Verification items for the finished model (mm, model axes). Face numbers are marked on the shaded views. A direction names the side the tool comes from. Coordinates: 2 decimals unless noted, no trailing zeros. Write each loop counter-clockwise with the first axis right and the second up, starting at its lowest first coordinate (ties: lowest second). Pieces come first, ordered by that corner, then holes. Notation, with made-up numbers: (38, -4) -> (50, -4) arc R25 ccw to (50, 8) -> close; hole circle Ø4 at (48.25, 9). An arc over 180 degrees is marked (long way). Write each question's results on one line, items separated by ' | '. Start each with the question number.
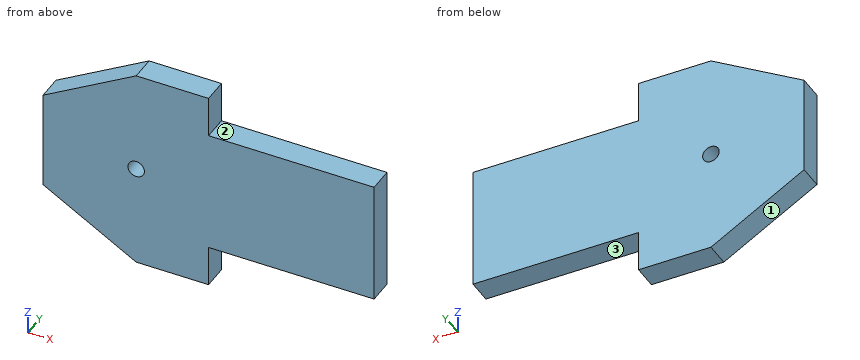
from build123d import *

# Parameters (mm, degrees)
BOSS_EXTRUDE1_DEPTH = 3
SKETCH2_R           = 1
CUT_EXTRUDE1_DEPTH  = 33


with BuildPart() as part:
    # Sketch1 → Boss-Extrude1 (new body)
    with BuildSketch(Plane(origin=(0, 0, 0), x_dir=(1, 0, 0), z_dir=(0, 1, 0))):
        Polygon((-10, 7.5), (-10, 12.5), (-18.741669751, 12.5), (-30, 6), (-30, -6), (-18.741669751, -12.5), (-10, -12.5), (-10, -7.5), (10, -7.5), (10, 7.5), align=None)
    extrude(amount=BOSS_EXTRUDE1_DEPTH)

    # Sketch2 → Cut-Extrude1 (cut)
    with BuildSketch(Plane(origin=(0, 3, 0), x_dir=(1, 0, 0), z_dir=(0, 1, 0))):
        with Locations(Location((-18.741669751, 0, 0), (0, 0, 270))):
            Circle(SKETCH2_R)
    extrude(amount=-CUT_EXTRUDE1_DEPTH, mode=Mode.SUBTRACT)


solid = part.part
1. Depth check by flat-ended pin: pin 1 Ø1.5 at (x, z) = (-5.5, -8.5) entering from +Y; pin 2 Ø1.5 at (y, z) = (1, -9.5) entering from +X; pin 3 Ø0.9 at (x, y) = (1.5, 2) entering from -Z. Enter the tip coordinate at first touch or a pass-through.
2. Material ranges on probe 1 along X at (y, z) = (1.3, 0); probe 2 along Z at (x, y) = (6.5, 1.2); probe 3 along X at (y, z) = (2.4, 8.75), recorded low to high. Write a range as from..to.
3. Sectioned sample at C-C on x = 4.5. Record the cut outline in (y, z), plus the area to 3 significant figures.
4. Sectioned sample at A-A on y = 1.7. Record the cut outline in (x, z), plus the area to 3 significant figures.
5. Tool access check on the marked faces 1, 2 and 3. Record the directions out of +Z, -Z, +X, -X, +Y, -Y that give a thin tool (end or side, any length) a straight path to the whole face; none if there is none.
6. Sectioned sample at D-D on x = -21. Record the cut outline in (y, z).
7. Sectioned sample at B-B on z = 0. Record the cut outline in (x, y), plus the area to 3 significant figures.
Computed values:
1) pin 1: passes through | pin 2: stops at x = -10 | pin 3: stops at z = -7.5
2) probe 1: x = -30..-19.74, -17.74..10 | probe 2: z = -7.5..7.5 | probe 3: x = -25.24..-10
3) outline: (0, -7.5) -> (3, -7.5) -> (3, 7.5) -> (0, 7.5) -> close | area: 45.0 mm^2
4) outline: (-30, -6) -> (-18.74, -12.5) -> (-10, -12.5) -> (-10, -7.5) -> (10, -7.5) -> (10, 7.5) -> (-10, 7.5) -> (-10, 12.5) -> (-18.74, 12.5) -> (-30, 6) -> close; hole circle Ø2 at (-18.74, 0) | area: 724 mm^2
5) face 1: -Z, -X, +Y, -Y | face 2: +Z, +X, +Y, -Y | face 3: -Z, +X, +Y, -Y
6) outline: (0, -11.2) -> (3, -11.2) -> (3, 11.2) -> (0, 11.2) -> close
7) outline: (-30, 0) -> (-19.74, 0) -> (-19.74, 3) -> (-30, 3) -> close; (-17.74, 0) -> (10, 0) -> (10, 3) -> (-17.74, 3) -> close | area: 114 mm^2
